Build history of the part. All positions in model axes, mm. A direction names the side the tool comes from. Coordinates: 2 decimals unless noted, no trailing zeros. Order: outer loops, then holes, each group sorted by start corner. A loop starts at its lowest first (then second) coordinate and runs counter-clockwise, first axis right, second up. Notation, with made-up numbers: (60.5, 51.5) - (98.5, 51.5) arc R16 ccw to (98.5, 65.5) - close; hole circle Ø5 at (-13, -31). An arc over 180 degrees is marked (long way). One line per item, written item: value.
from build123d import *

# Parameters (mm, degrees)
BOSS_EXTRUDE1_DEPTH      = 20.6375
BOSS_EXTRUDE1_DEPTH_BACK = 19.05
SKETCH3_W                = 149.554059724
SKETCH3_H                = 74.48224525
CUT_EXTRUDE1_DEPTH       = 516.127884509


with BuildPart() as part:
    # Sketch1 → Boss-Extrude1 (new, two sides: drawn at the far end of the back side and taken through both)
    with BuildSketch(Plane.XY.offset(-BOSS_EXTRUDE1_DEPTH_BACK)):
        with BuildLine():
            Line((357.059535637, 173.035014711), (357.059535637, 163.261817954))
            ThreePointArc((357.059535637, 163.261817954), (357.244928479, 162.517337083), (357.75780558, 161.946741471))
            Line((357.75780558, 161.946741471), (410.584136752, 126.226566951))
            Line((410.584136752, 126.226566951), (439.063985597, 126.226566951))
            Line((439.063985597, 126.226566951), (444.978063494, 141.390869249))
            Line((444.978063494, 141.390869249), (478.819933038, 133.446768417))
            ThreePointArc((478.819933038, 133.446768417), (479.648013751, 133.474476416), (480.349350513, 133.915625085))
            Line((480.349350513, 133.915625085), (484.344651115, 138.244883468))
            ThreePointArc((484.344651115, 138.244883468), (484.754953748, 139.504412771), (484.067254744, 140.636593142))
            Line((484.067254744, 140.636593142), (457.603933076, 158.530595004))
            Line((457.603933076, 158.530595004), (396.440312316, 158.530595004))
            Line((396.440312316, 158.530595004), (357.059535637, 173.035014711))
        make_face()
    extrude(amount=BOSS_EXTRUDE1_DEPTH + BOSS_EXTRUDE1_DEPTH_BACK)

    # Sketch3 → Cut-Extrude1 (cut, through all)
    with BuildSketch(Plane(origin=(0, 0.377817836, -2.785049831), x_dir=(1, 0, 0), z_dir=(0, -0.13442794428844543, 0.9909233713029392))):
        with Locations((424.804234836, 142.512706275)):
            Rectangle(SKETCH3_W, SKETCH3_H)
    extrude(amount=CUT_EXTRUDE1_DEPTH, mode=Mode.SUBTRACT)


solid = part.part
1. Band-saw the part on C-C, the plane x = 437.5. Give the cut face in (y, z).
Values found:
outline: (126.23, -19.05) - (158.53, -19.05) - (158.53, 18.67) - (126.23, 14.29) - close
2. Probe line 1 along Y through (x, z) = (416, 3); line 2 along X through (y, z) = (141.5, 10.5); line 3 along X through (y, z) = (149, -7). List the from-to ranges inside material, lowest first.
Values found:
line 1: y = 126.23 to 158.53
line 2: x = 388 to 482.79
line 3: x = 376.9 to 471.7
3. Two-plate mould, pull along X, no slides. Class faces 1 (the face through (441.98, 133.7, -1.6)), 2 (the face through (471.02, 149.46, -0.45)), 3 (the face through (420.02, 144.76, 16.8)): pulls with the +X half, pulls with the -X half, needs draft (parallel to the pull), parting line crosses it, or undercut.
Values found:
face 1: undercut
face 2: pulls with the +X half
face 3: needs draft
4. Band-saw the part on B-B, the plane z = -6. Give the cut face in (x, y) (1 decimal), and give its area (3 significant figures).
Values found:
outline: (357.1, 163.3) arc R1.6 ccw to (357.8, 161.9) - (410.6, 126.2) - (439.1, 126.2) - (445, 141.4) - (478.8, 133.4) arc R1.6 ccw to (480.3, 133.9) - (484.3, 138.2) arc R1.6 ccw to (484.1, 140.6) - (457.6, 158.5) - (396.4, 158.5) - (357.1, 173) - close
area: 2,710 mm2
5. 3-axis set-ups, long thin cutter, end or side, ignore diameter. For faces 4 (the face through (427, 158.531, 0)), 5 (the face through (461.662, 137.474, -1.6)), 6 (the face through (482.32, 136.05, -1.81)): which of +Z, -Z, +X, -X, +Y, -Y reach the whole face in a straight line?
Values found:
face 4: +Z, -Z, +X, +Y
face 5: +Z, -Z, -Y
face 6: +Z, -Z, +X, -Y
6. Flat gauge pins, fed straight in: P1, Ø1, axis at x = 471.5, z = -7.5, coming from the -Y side; P2, Ø5, axis at x = 387, z = 5, coming from the -Y side; P3, Ø4, axis at x = 384.5, z = 13.5, coming from the -Y side; P4, Ø10, axis at y = 162, z = -0.5, coming from the -X side. Where does each tip first touch, or does it go through?
Values found:
P1: stops at y = 135.05
P2: stops at y = 140.48
P3: stops at y = 142.51
P4: stops at x = 357.06
7. Band-saw the part on D-D, the plane y = 156.5. Give the cut face in (x, z).
Values found:
outline: (365.81, -19.05) - (460.61, -19.05) - (460.61, 18.39) - (365.81, 18.39) - close
8. Band-saw the part on A-A, the plane y = 139.5. Give the cut face in (x, z).
Values found:
outline: (390.95, -19.05) - (444.24, -19.05) - (444.24, 16.09) - (390.95, 16.09) - close; (453.03, -19.05) - (484.76, -19.05) - (484.76, 16.09) - (453.03, 16.09) - close
